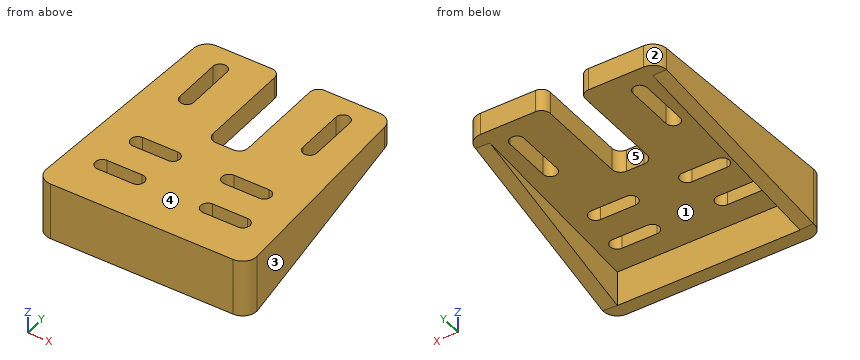
```python
from build123d import *

# Parameters (mm, degrees)
F1_DEPTH = 6.35
F3_DEPTH = 10
F4_SIZE2 = 9.99999
F4_SIZE  = 57.99999
F5_SIZE2 = 9.99999
F5_SIZE  = 57.99999


# Not quite as in the source:
# - a fillet or chamfer is up to 0.001 mm smaller than in the source, because OpenCascade refuses the exact size


with BuildPart() as f1:
    # F0 (on Top) → F1 (new body)
    with BuildSketch(Plane.XY):
        with BuildLine():
            Line((-26.0047037435, 0), (0, 0))
            Line((0, 0), (26.0047037435, 0))
            ThreePointArc((26.0047037435, 0), (28.9008830765, 1.2409883525), (30, 4.1939273644))
            Line((30, 4.1939273644), (27.1847426542, 62.1939273644))
            ThreePointArc((27.1847426542, 62.1939273644), (25.9484580453, 64.896179333), (23.1894463977, 66))
            Line((23.1894463977, 66), (7.5, 66))
            ThreePointArc((7.5, 66), (5.732233047, 65.267766953), (5, 63.5))
            Line((5, 63.5), (5, 37.5))
            ThreePointArc((5, 37.5), (4.267766953, 35.732233047), (2.5, 35))
            Line((2.5, 35), (0, 35))
            Line((0, 35), (-2.5, 35))
            ThreePointArc((-2.5, 35), (-4.267766953, 35.732233047), (-5, 37.5))
            Line((-5, 37.5), (-5, 63.5))
            ThreePointArc((-5, 63.5), (-5.732233047, 65.267766953), (-7.5, 66))
            Line((-7.5, 66), (-23.1894463977, 66))
            ThreePointArc((-23.1894463977, 66), (-25.9484580453, 64.896179333), (-27.1847426542, 62.1939273644))
            Line((-27.1847426542, 62.1939273644), (-30, 4.1939273644))
            ThreePointArc((-30, 4.1939273644), (-28.9008830765, 1.2409883525), (-26.0047037435, 0))
        make_face()
        with BuildLine():
            ThreePointArc((-20, 11), (-22, 13), (-20, 15))
            Line((-20, 15), (-10, 15))
            ThreePointArc((-10, 15), (-8, 13), (-10, 11))
            Line((-10, 11), (-20, 11))
        make_face(mode=Mode.SUBTRACT)
        with BuildLine():
            Line((-18, 27), (-8, 27))
            ThreePointArc((-8, 27), (-6, 25), (-8, 23))
            Line((-8, 23), (-18, 23))
            ThreePointArc((-18, 23), (-20, 25), (-18, 27))
        make_face(mode=Mode.SUBTRACT)
        with BuildLine():
            Line((10, 15), (20, 15))
            ThreePointArc((20, 15), (22, 13), (20, 11))
            Line((20, 11), (10, 11))
            ThreePointArc((10, 11), (8, 13), (10, 15))
        make_face(mode=Mode.SUBTRACT)
        with BuildLine():
            Line((18, 23), (8, 23))
            ThreePointArc((8, 23), (6, 25), (8, 27))
            Line((8, 27), (18, 27))
            ThreePointArc((18, 27), (20, 25), (18, 23))
        make_face(mode=Mode.SUBTRACT)
        with BuildLine():
            ThreePointArc((-15.5, 45), (-17.5, 43), (-19.5, 45))
            Line((-19.5, 45), (-19.5, 59))
            ThreePointArc((-19.5, 59), (-17.5, 61), (-15.5, 59))
            Line((-15.5, 59), (-15.5, 45))
        make_face(mode=Mode.SUBTRACT)
        with BuildLine():
            Line((15.5, 45), (15.5, 59))
            ThreePointArc((15.5, 59), (17.5, 61), (19.5, 59))
            Line((19.5, 59), (19.5, 45))
            ThreePointArc((19.5, 45), (17.5, 43), (15.5, 45))
        make_face(mode=Mode.SUBTRACT)
    extrude(amount=F1_DEPTH)

    # F2 (on face) → F3 (join)
    with BuildSketch(Plane.XY):
        with BuildLine():
            ThreePointArc((26.0047037435, 0), (28.9008830765, 1.2409883525), (30, 4.1939273644))
            Line((30, 4.1939273644), (26.0047037435, 4))
            Line((26.0047037435, 4), (-26.0047037435, 4))
            Line((-26.0047037435, 4), (-30, 4.1939273644))
            ThreePointArc((-30, 4.1939273644), (-28.9008830765, 1.2409883525), (-26.0047037435, 0))
            Line((-26.0047037435, 0), (0, 0))
            Line((0, 0), (26.0047037435, 0))
        make_face()
        Polygon((-30, 4.1939273644), (-26.0047037435, 4), (-23.1894463977, 62), (-27.1847426542, 62.1939273644), align=None)
        Polygon((26.0047037435, 4), (30, 4.1939273644), (27.1847426542, 62.1939273644), (23.1894463977, 62), align=None)
    extrude(amount=-F3_DEPTH)

    # F4 (size 58 and 10 in the source; OpenCascade refuses exactly that, so slightly less here)
    f4_edges = [f1.edges().sort_by_distance(p)[0] for p in [
        (-25.187095, 62.096964, -10),
    ]]
    f4_side = f1.faces().sort_by_distance((0, 0.864246, -10))[0]
    chamfer(f4_edges, length=F4_SIZE, length2=F4_SIZE2, reference=f4_side)

    # F5 (size 58 and 10 in the source; OpenCascade refuses exactly that, so slightly less here)
    f5_edges = [f1.edges().sort_by_distance(p)[0] for p in [
        (25.187095, 62.096964, -10),
    ]]
    f5_side = f1.faces().sort_by_distance((-25.139818, 3.992207, -10))[0]
    chamfer(f5_edges, length=F5_SIZE, length2=F5_SIZE2, reference=f5_side)


solid = f1.part
```
Source: CAD feature listing. Evaluate the final solid. Frame: model axes, mm. Face numbers are marked on the shaded views. A direction names the side the tool comes from. Round coordinates to 2 decimals unless told otherwise and drop trailing zeros. Loops run counter-clockwise (first coordinate to the right, second up) from the corner with the lowest first, then second, coordinate; pieces in that order, holes last.
(1) Contact query for flat-ended pins moving along their axis: pin 1 Ø5 at (x, z) = (-2, -4) entering from +Y; pin 2 Ø5 at (x, y) = (-8.5, 43.5) entering from -Z; pin 3 Ø7 at (y, z) = (51, 2) entering from +X. Output: stop coordinate, or through.
From the geometry:
pin 1: stops at y = 4
pin 2: stops at z = 0
pin 3: stops at x = 27.9
(2) Pull-direction query (X, two-part tool) for the marked faces 1, 2 and 3; classes: +X half, -X half, draft (parallel to the pull), parting line (faces both ways), or undercut.
From the geometry:
face 1: undercut
face 2: -X half
face 3: +X half
(3) Material intervals for probe 1 along X at (y, z) = (52.5, 3.75); probe 2 along Z at (x, y) = (22, 47); probe 3 along X at (y, z) = (10.5, -1), sorted ascending.
From the geometry:
probe 1: x = -27.66 to -19.5, -15.5 to -5, 5 to 15.5, 19.5 to 27.66
probe 2: z = 0 to 6.35
probe 3: x = -29.69 to -25.69, 25.69 to 29.69
(4) Section query C-C (y = 13.5). Output: boundary loops of the cut face in (x, z).
From the geometry:
outline: (-29.55, -8.41) - (-25.54, -8.37) - (-25.54, 0) - (-21.94, 0) - (-21.94, 6.35) - (-29.55, 6.35) - close; (-8.06, 0) - (8.06, 0) - (8.06, 6.35) - (-8.06, 6.35) - close; (21.94, 0) - (25.54, 0) - (25.54, -8.37) - (29.55, -8.41) - (29.55, 6.35) - (21.94, 6.35) - close
(5) Section query A-A (y = 51). Output: boundary loops of the cut face in (x, z).
From the geometry:
outline: (-27.73, -1.93) - (-23.72, -1.9) - (-23.72, 0) - (-19.5, 0) - (-19.5, 6.35) - (-27.73, 6.35) - close; (-15.5, 0) - (-5, 0) - (-5, 6.35) - (-15.5, 6.35) - close; (5, 0) - (15.5, 0) - (15.5, 6.35) - (5, 6.35) - close; (19.5, 0) - (23.72, 0) - (23.72, -1.9) - (27.73, -1.93) - (27.73, 6.35) - (19.5, 6.35) - close
(6) Section query D-D (z = 4.25). Give the number of separate pieces and of enclosed holes in the cut face, and give its area (3 significant figures).
From the geometry:
separate pieces: 1
enclosed holes: 6
area: 3,100 mm2
(7) Access query for the marked faces 4 and 5. Directions: +Z, -Z, +X, -X, +Y, -Y. A direction counts if a zero-diameter tool reaches every point of the face in a straight line with its end or side. Return the directions, or none.
From the geometry:
face 4: +Z, +X, -X, +Y, -Y
face 5: +Z, -Z, +Y
(8) Section query B-B (z = -5). Output: boundary loops of the cut face in (x, y), and give its area (3 significant figures).
From the geometry:
outline: (-30, 4.19) arc R4 ccw to (-26, 0) - (26, 0) arc R4 ccw to (30, 4.19) - (28.59, 33.23) - (24.6, 33.03) - (26, 4) - (-26, 4) - (-24.6, 33.03) - (-28.59, 33.23) - close
area: 466 mm2
